Verification items for the finished model (mm, model axes). Face numbers are marked on the shaded views. Give positions to 0.01 mm unless a question says otherwise; leave off trailing zeros. Order: outer loops, then holes, each group sorted by start corner. A loop starts at its lowest first (then second) coordinate and runs counter-clockwise, first axis right, second up. Notation, with made-up numbers: (52.25, 5.5) -> (91.25, 5.5) arc R33 cw to (91.25, 37.5) -> close; hole circle Ø4 at (86, 52.25). An arc over 180 degrees is marked (long way). One line per question, with ' | ' between items. Start each with the question number.
Q1. Section check C-C on z = 0. Record the cut outline in (x, y).
Q2. Material ranges on probe 1 along Z at (x, y) = (-29, 3.75); probe 2 along X at (y, z) = (4, -14); probe 3 along Y at (x, z) = (-2, 13.5), recorded low to high. Write a range as [from, to].
Q3. Section check A-A on x = 0. Give the number of separate pieces and of enclosed holes in the cut face, plus the area to 3 significant figures.
Q4. Section check B-B on y = 5.5. Record the cut outline in (x, z).
Q5. Go/stop test with flat-tipped pins: pin 1 (8 mm diameter, centred on y = 6.5, z = 22.5, fed in from -X); pin 2 (5.5 mm diameter, centred on x = 32, z = -17.5, fed in from -Y); pin 3 (9 mm diameter, centred on x = 0, z = 37.5, fed in from +Y); pin 4 (5 mm diameter, centred on x = 32.48, z = -18.75, fed in from -Y). Record where each tip stops, or that it passes through.
Q6. Mould release check, pull along X, two halves, no side actions. Record for the marked faces 1, 2 and 3: released by +X, released by -X, zero draft, split by the parting line, or undercut.
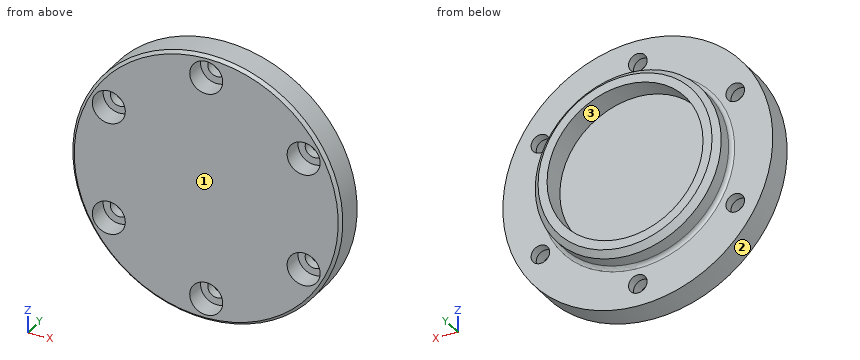
Autodesk Inventor part; units mm, degrees
ref_plane "YZ Plane" through (0, 0, 0) normal (1, 0, 0) x (0, 1, 0)
ref_plane "XZ Plane" through (0, 0, 0) normal (0, 1, 0) x (-1, 0, 0)
ref_plane "XY Plane" through (0, 0, 0) normal (0, 0, 1) x (1, 0, 0)
sketch "Эскиз1" plane through (0, 0, 0) normal (0, 0, 1) x (1, 0, 0)
  line L0 (0, 5) -> (0, 0)
  line L1 (0, 0) -> (31, 0)
  line L2 (31, 0) -> (31, 18)
  line L3 (31, 18) -> (26, 18)
  line L4 (26, 18) -> (26, 5)
  line L5 (26, 5) -> (0, 5)
  dimension "d0" = 18
  dimension "d1" = 5
  dimension "d3" = 31
revolve "Вращение1" add sketch "Эскиз1" angle 360 about axis through (0, 5, 0) along (0, -1, 0)
sketch "Эскиз2" plane through (0, 0, 0) normal (1, 0, 0) x (0, 1, 0)
  line L0 (0, 31) -> (0, -31)
  line L1 (18, 31) -> (0, 31)
  line L2 (18, 31) -> (0, 31)
  line L3 (0, 0) -> (0, 45)
  line L4 (0, 45) -> (10, 45)
  line L5 (10, 45) -> (10, 0)
  line L6 (10, 0) -> (0, 0)
  line L7 (-4.2, 0) -> (25.2, 0)
  dimension "d5" = 10
  dimension "d6" = 45
revolve "Вращение2" add sketch "Эскиз2" angle 360 about axis through (0, -10, 0) along (0, 1, 0)
sketch "Эскиз3" plane through (0, 0, 0) normal (0, -1, 0) x (1, 0, 0)
  line L0 (0, -63) -> (0, 63)
  line L1 (-63, 0) -> (63, 0)
  circle A0 centre (0, 0) radius 37.5 construction
  circle A1 centre (0, 37.5) radius 5.5
  dimension "d8" = 75
  dimension "d9" = 11
hole "Отверстие1" at (0, 0, 37.5) direction (0, 1, 0) diameter 6.2 depth 15 tip angle 118 counterbore diameter 11 counterbore depth 6.8
pattern_circular "Круговой массив1" count 6 over 360 about axis through (0, -10, 0) along (0, 1, 0) of "Отверстие1"
fillet "Сопряжение1" radius 1.3 1 edges at (-31, 10, 0)
chamfer "Фаска1" distance 1 angle 45 1 edges at (0, 0, -45)
chamfer "Фаска2" distance 2 angle 45 1 edges at (-31, 18, 0)
properties part number "Крышка маленькая_62"
Filled in:
1) outline: (-45, 1) -> (-44, 0) -> (44, 0) -> (45, 1) -> (45, 10) -> (32.3, 10) arc R1.3 cw to (31, 11.3) -> (31, 16) -> (29, 18) -> (26, 18) -> (26, 10) -> (-26, 10) -> (-26, 18) -> (-29, 18) -> (-31, 16) -> (-31, 11.3) arc R1.3 cw to (-32.3, 10) -> (-45, 10) -> close
2) probe 1: [-34.41, -23.01], [-14.49, 14.49], [23.01, 34.41] | probe 2: [-42.77, -35.25], [-29.7, 29.7], [35.25, 42.77] | probe 3: [0, 10]
3) separate pieces: 3 | enclosed holes: 0 | area: 786 mm²
4) outline: circle Ø90 at (0, 0); hole circle Ø11 at (-32.48, -18.75); hole circle Ø11 at (-32.48, 18.75); hole circle Ø11 at (0, -37.5); hole circle Ø11 at (0, 37.5); hole circle Ø11 at (32.48, -18.75); hole circle Ø11 at (32.48, 18.75)
5) pin 1: x = -41.02 | pin 2: y = 6.8 | pin 3: y = 10 | pin 4: through
6) face 1: zero draft | face 2: split by the parting line | face 3: undercut
